Could you check a few things on this model? Use its own coordinates, in mm. Give positions to 0.01 mm unless a question says otherwise; leave off trailing zeros. Loops run counter-clockwise (first coordinate to the right, second up) from the corner with the lowest first, then second, coordinate; pieces in that order, holes last. Notation, with made-up numbers: M 33.25,22.25 L 56.25,22.25 A20 ccw 56.25,58.25 Z; hole C -33.5,-15 d8. An arc over 180 degrees is marked long. Use CSV: the item, a comma, the result in double quotes.
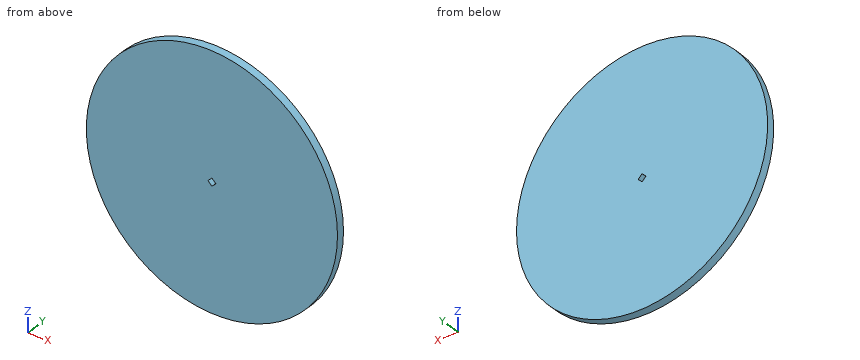
```python
from build123d import *

# Parameters (mm, degrees)
F0_R     = 50.8
F1_DEPTH = 3.175


with BuildPart() as f1:
    # F0 (on Front) → F1 (new body)
    with BuildSketch(Plane.XZ):
        Circle(F0_R)
        Polygon((-1.5875, 0), (0, 1.5875), (1.5875, 0), (0, -1.5875), align=None, mode=Mode.SUBTRACT)
    extrude(amount=F1_DEPTH)


solid = f1.part
```
1. I want a section at C-C, the plane x = -44. List the corners of the cut face in (y, z) for me (3 decimals), then the cut area to 3 significant figures.
Outcome:
outline,"M -3.175,-25.39 L 0,-25.39 L 0,25.39 L -3.175,25.39 Z"
area,"161 mm2"
2. I want a section at A-A, the plane y = -1.4. List the corners of the cut face in (x, z) for me.
Outcome:
outline,"C 0,0 d101.6; hole M -1.59,0 L 0,-1.59 L 1.59,0 L 0,1.59 Z"
3. Please list where these lines run through material, in increasing order: line 1 (X direction, y = -1.6, z = 1); line 2 (Z direction, x = 21.5, y = -1.15); line 3 (X direction, y = -2.7, z = -42.5).
Outcome:
line 1,"-50.79 to -0.59, 0.59 to 50.79"
line 2,"-46.03 to 46.03"
line 3,"-27.83 to 27.83"
4. I want a section at B-B, the plane z = -37. List the corners of the cut face in (x, y) for me (3 decimals).
Outcome:
outline,"M -34.809,-3.175 L 34.809,-3.175 L 34.809,0 L -34.809,0 Z"
5. I'm going to push a flat-ended pin straight in: pin 1 Ø1.5 at (x, y) = (-1, -2.5) entering from +Z. Where does the tip first touch, or does it pass through?
Outcome:
pin 1,"z = 50.8"
